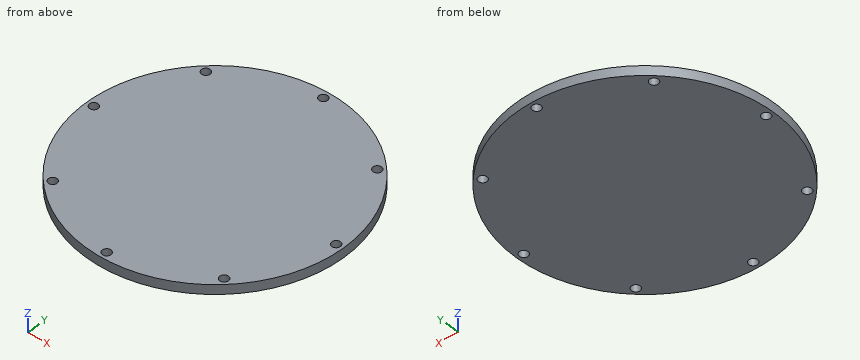
```python
from build123d import *

# Parameters (mm, degrees)
SKETCH1_R                      = 75.565
BOSS_EXTRUDE1_DEPTH            = 5.6
F_8_0_199_DIAMETER_HOLE1_D     = 5.0546
F_8_0_199_DIAMETER_HOLE1_DEPTH = 8.481444958
F_8_0_199_DIAMETER_HOLE1_TIP   = 1.518555042


with BuildPart() as part:
    # Sketch1 → Boss-Extrude1 (new body)
    with BuildSketch(Plane.XY):
        Circle(SKETCH1_R)
    extrude(amount=BOSS_EXTRUDE1_DEPTH)

    # #8 (0.199) Diameter Hole1
    with Locations(Plane(origin=(0, 0, 0), x_dir=(-1, 0, 0), z_dir=(0, 0, -1))):
        with Locations((-50.478019657, 50.478019657), (0, 71.3867), (50.478019657, 50.478019657), (71.3867, 0), (50.478019657, -50.478019657), (0, -71.3867), (-50.478019657, -50.478019657), (-71.3867, 0)):
            Hole(F_8_0_199_DIAMETER_HOLE1_D / 2, depth=F_8_0_199_DIAMETER_HOLE1_DEPTH)
            with Locations((0, 0, -(F_8_0_199_DIAMETER_HOLE1_DEPTH + F_8_0_199_DIAMETER_HOLE1_TIP / 2))):  # 118° drill point
                Cone(0, F_8_0_199_DIAMETER_HOLE1_D / 2, F_8_0_199_DIAMETER_HOLE1_TIP, mode=Mode.SUBTRACT)


solid = part.part
```
Input: part model. Units: mm. Frame: model coordinates. Give positions to 0.01 mm unless a question says otherwise; leave off trailing zeros. Order: outer loops, then holes, each group sorted by start corner. A loop starts at its lowest first (then second) coordinate and runs counter-clockwise, first axis right, second up.
1. Section C-C on z = 1.4. Give the number of separate pieces and of enclosed holes in the cut face, and give its area (3 significant figures).
Derived:
separate pieces: 1
enclosed holes: 8
area: 17,800 mm2
2. Material intervals for L1, parallel to Y at x = 0, z = 1.5 (3 decimals); L2, parallel to Y at x = -50.5, z = 0.9; L3, parallel to Y at x = 7, z = 3.55, sorted ascending.
Derived:
L1: y = -75.565 to -73.914, -68.859 to 68.859, 73.914 to 75.565
L2: y = -56.21 to -53.01, -47.95 to 47.95, 53.01 to 56.21
L3: y = -75.24 to 75.24
3. Section A-A on y = 0. Return the cut outline in (x, z) (3 decimals).
Derived:
outline: (-75.565, 0) - (-73.914, 0) - (-73.914, 5.6) - (-75.565, 5.6) - close; (-68.859, 0) - (68.859, 0) - (68.859, 5.6) - (-68.859, 5.6) - close; (73.914, 0) - (75.565, 0) - (75.565, 5.6) - (73.914, 5.6) - close
4. Section D-D on y = 19. Return the cut outline in (x, z), and give its area (3 significant figures).
Derived:
outline: (-73.14, 0) - (73.14, 0) - (73.14, 5.6) - (-73.14, 5.6) - close
area: 819 mm2
5. Pin query (flat end, axial travel): pin 1 (2 mm diameter, centred on y = 28.5, z = 1, fed in from +X); pin 2 (4 mm diameter, centred on x = -50.48, y = 50.48, fed in from +Z); pin 3 (1 mm diameter, centred on y = -51, z = 3, fed in from -X); pin 4 (3 mm diameter, centred on x = -49, z = 2.5, fed in from +Y). Return the tip coordinate at first contact, or that it passes through.
Derived:
pin 1: stops at x = 70.38
pin 2: passes through
pin 3: stops at x = -56.21
pin 4: stops at y = 58.77
